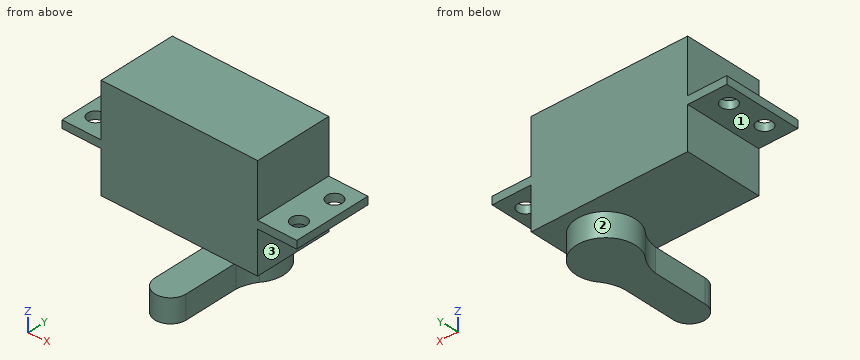
Autodesk Inventor part; units mm, degrees
ref_plane "Work Plane1" through (20, 0, -42.5) normal (0, 0, -1) x (-1, 0, 0)
ref_plane "YZ Plane" through (0, 0, 0) normal (1, 0, 0) x (0, 1, 0)
ref_plane "XZ Plane" through (0, 0, 0) normal (0, 1, 0) x (-1, 0, 0)
sketch "Sketch1" plane through (0, 0, 0) normal (0, 1, 0) x (-1, 0, 0)
  line L0 (-20, 0) -> (20, 0)
  line L1 (20, 0) -> (20, -40.5)
  line L2 (20, -40.5) -> (-20, -40.5)
  line L3 (-20, -40.5) -> (-20, 0)
  point P0 (0, 0)
  point P1 (0, -40.5)
  dimension "d0" = 40
  dimension "d1" = 40.5
extrude "Extrusion1" add sketch "Sketch1" along normal blind 20
sketch "Sketch2" plane through (20, 0, 0) normal (1, 0, 0) x (0, 0, -1)
  line L0 (27.7, 20) -> (29.7, 20)
  line L1 (29.7, 20) -> (29.7, 0)
  line L2 (29.7, 0) -> (27.7, 0)
  line L3 (27.7, 0) -> (27.7, 20)
  line L4 (40.5, 0) -> (40.5, 20)
  line L5 (0, 0) -> (0, 20)
  dimension "d4" = 2
  dimension "d31" = 27.7
extrude "Extrusion2" add sketch "Sketch2" along normal blind 10
sketch "Sketch3" plane through (20, 0, -29.7) normal (0, 0, -1) x (-1, 0, 0)
  circle A0 centre (-6, 15) radius 2
  line L0 (-10, 20) -> (-10, 0)
  line L1 (-10, 10) -> (0, 10)
  circle A1 centre (-6, 5) radius 2
  point P0 (20, 0)
  point P1 (-8, 6.7321)
  point P2 (-8, 3.2679)
  dimension "d9" = 4
  dimension "d13" = 5
  dimension "d33" = 4
extrude "Extrusion3" cut sketch "Sketch3" against normal up to next
sketch "Sketch4" plane through (20, 0, -40.5) normal (0, 0, -1) x (-1, 0, 0)
  circle A0 centre (10, 10) radius 3
  line L0 (0, 0) -> (0, 20)
  line L1 (0, 20) -> (40, 20)
  point P0 (20, 0)
  dimension "d16" = 6
  dimension "d17" = 10
  dimension "d18" = 10
extrude "Extrusion4" add sketch "Sketch4" along normal blind 6
mirror "Mirror1" about plane through (0, 0, 0) normal (1, 0, 0) of "Extrusion2", "Extrusion3"
ref_plane "Work Plane1" through (20, 0, -42.5) normal (0, 0, -1) x (-1, 0, 0)
sketch "Sketch6" plane through (20, 0, -40.5) normal (0, 0, -1) x (-1, 0, 0)
  line L0 (6, 0.4936) -> (6, -13.5)
  arc A0 (6, -13.5) -> (14, -13.5) centre (10, -13.5) ccw
  line L1 (14, -13.5) -> (14, 0.4936)
  arc A1 (15.7453, 5.1791) -> (14, 0.4936) centre (23.9461, -0.5435) ccw
  arc A2 (15.7453, 5.1791) -> (4.2547, 5.1791) centre (10, 10) ccw
  arc A3 (6, 0.4936) -> (4.2547, 5.1791) centre (-3.9461, -0.5435) ccw
  line L2 (14.2, 0.4832) -> (14.2, -13.5)
  arc A4 (5.8, -13.5) -> (14.2, -13.5) centre (10, -13.5) ccw
  line L3 (5.8, -13.5) -> (5.8, 0.4832)
  arc A5 (5.8, 0.4832) -> (4.0957, 5.0574) centre (-3.9461, -0.5435) ccw
  arc A6 (15.9043, 5.0574) -> (4.0957, 5.0574) centre (10, 10) ccw
  arc A7 (15.9043, 5.0574) -> (14.2, 0.4832) centre (23.9461, -0.5435) ccw
  circle A8 centre (10, 10) radius 3
  point P0 (20, 0)
  dimension "d35" = 0.2
extrude "Extrusion6" add sketch "Sketch6" along normal blind 6 contours A3 A2 A1 L1 A0 L0
sketch "Sketch7" plane through (-20, 0, 0) normal (0, 0, 1) x (1, 0, 0)
  line L0 (0, 0) -> (40, 0)
  line L1 (40, 0) -> (40, 20)
  line L2 (0, 20) -> (40, 20)
  line L3 (0, 0) -> (0, 20)
  point P0 (20, 0)
extrude "Extrusion7" cut sketch "Sketch7" against normal blind 14
properties part number "Servo" material "PLA"
Here's how the part is built. I have some questions about the finished solid (model axes, mm). Face numbers are marked on the shaded views. A direction names the side the tool comes from. Give positions to 0.01 mm unless a question says otherwise; leave off trailing zeros. Loops run counter-clockwise (first coordinate to the right, second up) from the corner with the lowest first, then second, coordinate; pieces in that order, holes last. Notation, with made-up numbers: (51, 1.5) -> (91, 1.5) arc R13 cw to (91, 12.5) -> close; hole circle Ø5 at (63, 48.25). An arc over 180 degrees is marked (long way). Use one line per item in the form item = value. Start each with the question number.
1) Please list where these lines run through material, in increasing order: line 1 along Y through (x, z) = (26, -28); line 2 along X through (y, z) = (14, -34); line 3 along Y through (x, z) = (19.5, -28).
2) Imagine slicing it at B-B (x = 10). Please give me the cut outline in (y, z).
3) Imagine slicing it at D-D (y = 10). Please give me the cut outline in (x, z), then the cut area to 3 significant figures.
4) Which directions (+Z, -Z, +X, -X, +Y, -Y) give clear straight access to the entire face, cutting with the end or side of a thin tool? Please do the marked faces 1, 2 and 3.
5) For P1, Ø8, axis at x = -2.5, z = -22.5, coming from the -Y side; P2, Ø6, axis at y = 9, z = -24.5, coming from the -X side; P3, Ø4.5, axis at x = -26, y = 5, coming from the -Z side, each with a flat end and sliding along its axis, tell me the tip position at first contact or that it passes through.
6) Imagine slicing it at C-C (y = 15). Please give me the cut outline in (x, z).
7) Imagine slicing it at A-A (x = 26). Please give me the cut outline in (y, z).
Check values:
q1.line_1 = 0 to 3, 7 to 13, 17 to 20
q1.line_2 = -20 to 20
q1.line_3 = 0 to 20
q2.outline = (-17.5, -46.5) -> (17.5, -46.5) -> (17.5, -40.5) -> (20, -40.5) -> (20, -14) -> (0, -14) -> (0, -40.5) -> (-17.5, -40.5) -> close
q3.outline = (-30, -29.7) -> (-20, -29.7) -> (-20, -40.5) -> (2.5, -40.5) -> (2.5, -46.5) -> (17.5, -46.5) -> (17.5, -40.5) -> (20, -40.5) -> (20, -29.7) -> (30, -29.7) -> (30, -27.7) -> (20, -27.7) -> (20, -14) -> (-20, -14) -> (-20, -27.7) -> (-30, -27.7) -> close
q3.area = 1,190 mm^2
q4.face_1 = -Z, -X, +Y, -Y
q4.face_2 = -Z
q4.face_3 = -Z, +X, +Y, -Y
q5.P1 = 0
q5.P2 = -20
q5.P3 = -29.7
q6.outline = (-30, -29.7) -> (-28, -29.7) -> (-28, -27.7) -> (-30, -27.7) -> close; (-24, -29.7) -> (-20, -29.7) -> (-20, -40.5) -> (4.41, -40.5) -> (4.41, -46.5) -> (15.59, -46.5) -> (15.59, -40.5) -> (20, -40.5) -> (20, -29.7) -> (24, -29.7) -> (24, -27.7) -> (20, -27.7) -> (20, -14) -> (-20, -14) -> (-20, -27.7) -> (-24, -27.7) -> close; (28, -29.7) -> (30, -29.7) -> (30, -27.7) -> (28, -27.7) -> close
q7.outline = (0, -29.7) -> (3, -29.7) -> (3, -27.7) -> (0, -27.7) -> close; (7, -29.7) -> (13, -29.7) -> (13, -27.7) -> (7, -27.7) -> close; (17, -29.7) -> (20, -29.7) -> (20, -27.7) -> (17, -27.7) -> close
